from build123d import *

# Parameters (mm, degrees)
BOSS_EXTRUDE1_DEPTH = 2.5
CUT_EXTRUDE1_REACH  = 26.645
SKETCH2_R           = 1.715
SKETCH2_R_2         = 8.98
SKETCH3_R           = 2.6543
BOSS_EXTRUDE2_DEPTH = 70.305
BOSS_EXTRUDE3_START = 4
SKETCH4_R           = 21
SKETCH4_R_2         = 8.98
BOSS_EXTRUDE3_DEPTH = 4
SKETCH6_R           = 21
SKETCH6_R_2         = 8.98
BOSS_EXTRUDE4_DEPTH = 2
CUT_EXTRUDE3_START  = -15
SKETCH7_R           = 1.715
CUT_EXTRUDE3_DEPTH  = 15
SKETCH8_R           = 8.98
CUT_EXTRUDE4_DEPTH  = 2
SKETCH9_R           = 11.0744
SKETCH9_R_2         = 8.98
BOSS_EXTRUDE5_DEPTH = 2.35
BOSS_EXTRUDE6_REACH = 82.451
SKETCH10_R          = 12.48
SKETCH10_R_2        = 8.98
SKETCH12_R          = 21
SKETCH12_R_2        = 12.48
CUT_EXTRUDE5_DEPTH  = 57.805


with BuildPart() as part:
    # Sketch1 → Boss-Extrude1 (new body)
    with BuildSketch(Plane(origin=(0, 0, 0), x_dir=(1, 0, 0), z_dir=(0, 1, 0))):
        with BuildLine():
            Line((0.597960958, 12.236443242), (0.597960958, 17.5133))
            Line((0.597960958, 17.5133), (-2.819411684, 17.5133))
            Line((-2.819411684, 17.5133), (-2.819411684, 11.976881697))
            ThreePointArc((-2.819411684, 11.976881697), (-9.752212861, 8.278991937), (-13.533031252, 1.391065316))
            ThreePointArc((-13.533031252, 1.391065316), (-17.156497956, -0.999626805), (-13.683409812, -3.603965207))
            ThreePointArc((-13.683409812, -3.603965207), (-10.042516815, -11.01106651), (-2.819411684, -15.004561697))
            Line((-2.819411684, -15.004561697), (-2.819411684, -17.5133))
            Line((-2.819411684, -17.5133), (0.597960958, -17.5133))
            Line((0.597960958, -17.5133), (0.597960958, -15.264123242))
            ThreePointArc((0.597960958, -15.264123242), (9.161591247, -11.721092084), (13.538839655, -3.55233882))
            ThreePointArc((13.538839655, -3.55233882), (17.156522938, -1.000460972), (13.393344487, 1.331534062))
            ThreePointArc((13.393344487, 1.331534062), (8.853545908, 8.96396608), (0.597960958, 12.236443242))
        make_face()
    extrude(amount=BOSS_EXTRUDE1_DEPTH)

    # Sketch2 → Cut-Extrude1 (cut, up to next)
    with BuildSketch(Plane(origin=(0, 2.5, 0), x_dir=(1, 0, 0), z_dir=(0, 1, 0)), mode=Mode.PRIVATE) as cut_extrude1_sk1:
        with Locations(Location((-14.5034, -1.0795, 0), (0, 0, 270))):
            Circle(SKETCH2_R)
    cut_extrude1_tool1 = extrude(cut_extrude1_sk1.sketch, amount=-CUT_EXTRUDE1_REACH, mode=Mode.PRIVATE) & part.part
    # Sketch2 → Cut-Extrude1 (cut, up to next)
    with BuildSketch(Plane(origin=(0, 2.5, 0), x_dir=(1, 0, 0), z_dir=(0, 1, 0)), mode=Mode.PRIVATE) as cut_extrude1_sk2:
        with Locations(Location((14.5034, -1.0795, 0), (0, 0, 270))):
            Circle(SKETCH2_R)
    cut_extrude1_tool2 = extrude(cut_extrude1_sk2.sketch, amount=-CUT_EXTRUDE1_REACH, mode=Mode.PRIVATE) & part.part
    # Sketch2 → Cut-Extrude1 (cut, up to next)
    with BuildSketch(Plane(origin=(0, 2.5, 0), x_dir=(1, 0, 0), z_dir=(0, 1, 0)), mode=Mode.PRIVATE) as cut_extrude1_sk3:
        with Locations(Location((-0.0762, -1.51384, 0), (0, 0, 270))):
            Circle(SKETCH2_R_2)
    cut_extrude1_tool3 = extrude(cut_extrude1_sk3.sketch, amount=-CUT_EXTRUDE1_REACH, mode=Mode.PRIVATE) & part.part
    add(cut_extrude1_tool1.solids().sort_by_distance((-14.5034, 2.5, 1.0795))[0], mode=Mode.SUBTRACT)
    add(cut_extrude1_tool2.solids().sort_by_distance((14.5034, 2.5, 1.0795))[0], mode=Mode.SUBTRACT)
    add(cut_extrude1_tool3.solids().sort_by_distance((-0.0762, 2.5, 1.51384))[0], mode=Mode.SUBTRACT)

    # Sketch3 → Boss-Extrude2 (add)
    with BuildSketch(Plane(origin=(0, 2.5, 0), x_dir=(1, 0, 0), z_dir=(0, 1, 0))):
        with Locations(Location((-14.5034, -1.0795, 0), (0, 0, 68.556492541))):
            Circle(SKETCH3_R)
        with Locations(Location((14.5034, -1.0795, 0), (0, 0, 114.72164566))):
            Circle(SKETCH3_R)
    extrude(amount=BOSS_EXTRUDE2_DEPTH)

    # Sketch4 → Boss-Extrude3 (add)
    with BuildSketch(Plane(origin=(0, 72.805, 0), x_dir=(1, 0, 0), z_dir=(0, 1, 0)).offset(BOSS_EXTRUDE3_START)):
        with Locations(Location((-0.0762, -1.51384, 0), (0, 0, 270))):
            Circle(SKETCH4_R)
        with Locations(Location((-0.0762, -1.51384, 0), (0, 0, 270))):
            Circle(SKETCH4_R_2, mode=Mode.SUBTRACT)
    extrude(amount=-BOSS_EXTRUDE3_DEPTH)

    # Sketch6 → Boss-Extrude4 (add)
    with BuildSketch(Plane(origin=(0, 37.805, 0), x_dir=(-1, 0, 0), z_dir=(0, -1, 0))):
        with Locations(Location((0.0762, -1.51384, 0), (0, 0, 90))):
            Circle(SKETCH6_R)
        with Locations(Location((0.0762, -1.51384, 0), (0, 0, 270))):
            Circle(SKETCH6_R_2, mode=Mode.SUBTRACT)
    extrude(amount=BOSS_EXTRUDE4_DEPTH)

    # Sketch7 → Cut-Extrude3 (cut)
    with BuildSketch(Plane.XZ.offset(CUT_EXTRUDE3_START)):
        with Locations(Location((-14.5034, 1.0795, 0), (0, 0, 90))):
            Circle(SKETCH7_R)
        with Locations(Location((14.5034, 1.0795, 0), (0, 0, 90))):
            Circle(SKETCH7_R)
    extrude(amount=CUT_EXTRUDE3_DEPTH, mode=Mode.SUBTRACT)

    # Sketch8 → Cut-Extrude4 (cut)
    with BuildSketch(Plane(origin=(0, 76.805, 0), x_dir=(1, 0, 0), z_dir=(0, 1, 0))):
        with BuildLine():
            Line((-10.0762, -1.51384), (-7.3262, -15.51384))
            ThreePointArc((-7.3262, -15.51384), (-0.0762, -17.51384), (7.1738, -15.51384))
            Line((7.1738, -15.51384), (9.9238, -1.51384))
            Line((9.9238, -1.51384), (7.1738, 12.48616))
            ThreePointArc((7.1738, 12.48616), (-0.0762, 14.48616), (-7.3262, 12.48616))
            Line((-7.3262, 12.48616), (-10.0762, -1.51384))
        make_face()
        with Locations(Location((-0.0762, -1.51384, 0), (0, 0, 270))):
            Circle(SKETCH8_R, mode=Mode.SUBTRACT)
    extrude(amount=-CUT_EXTRUDE4_DEPTH, mode=Mode.SUBTRACT)

    # Sketch9 → Boss-Extrude5 (add)
    with BuildSketch(Plane.XZ):
        with Locations(Location((-0.0762, 1.51384, 0), (0, 0, 90))):
            Circle(SKETCH9_R)
        with Locations(Location((-0.0762, 1.51384, 0), (0, 0, 90))):
            Circle(SKETCH9_R_2, mode=Mode.SUBTRACT)
    extrude(amount=BOSS_EXTRUDE5_DEPTH)

    # Boss-Extrude6: up to this face of the body (flat: up to its plane)
    boss_extrude6_end = Plane(part.part.faces().sort_by_distance((-0.0762, 72.805, -18.892190304))[0])
    # Sketch10 → Boss-Extrude6 (add, up to the picked face)
    with BuildSketch(Plane(origin=(0, 2.5, 0), x_dir=(1, 0, 0), z_dir=(0, 1, 0)), mode=Mode.PRIVATE) as boss_extrude6_sk1:
        with Locations((-0.0762, -1.51384)):
            Circle(SKETCH10_R)
        with Locations(Location((-0.0762, -1.51384, 0), (0, 0, 270))):
            Circle(SKETCH10_R_2, mode=Mode.SUBTRACT)
    boss_extrude6_tool1 = split(extrude(boss_extrude6_sk1.sketch, amount=BOSS_EXTRUDE6_REACH, mode=Mode.PRIVATE), bisect_by=boss_extrude6_end, keep=Keep.BOTH, mode=Mode.PRIVATE)
    add(boss_extrude6_tool1.solids().sort_by(Axis((-12.203212, 2.5, 1.51384), (0, 1, 0)))[0])

    # Sketch12 → Cut-Extrude5 (cut)
    with BuildSketch(Plane.XZ.offset(-15)):
        with Locations(Location((-0.0762, 1.51384, 0), (0, 0, 90))):
            Circle(SKETCH12_R)
        with Locations(Location((-0.0762, 1.51384, 0), (0, 0, 189.400360909))):
            Circle(SKETCH12_R_2, mode=Mode.SUBTRACT)
    extrude(amount=-CUT_EXTRUDE5_DEPTH, mode=Mode.SUBTRACT)


solid = part.part
Source: CAD feature listing. Evaluate the final solid. Frame: model axes, mm. A direction names the side the tool comes from. Give positions to 0.01 mm unless a question says otherwise; leave off trailing zeros. Write each loop counter-clockwise with the first axis right and the second up, starting at its lowest first coordinate (ties: lowest second). Pieces come first, ordered by that corner, then holes. Notation, with made-up numbers: M 63.25,59 L 90.25,59 A14 ccw 90.25,79 Z; hole C -36,47.5 d3. An arc over 180 degrees is marked long. Return JSON: item names as keys, results as strings. Group by question number.
1) Ray query, L1, parallel to Z at x = 0, y = 2; L2, parallel to Y at x = -11.5, z = 9 (3 decimals); L3, parallel to Y at x = 14.5, z = -0.5 (3 decimals). Return the intervals inside material, ascending.
2) Draft query along Z for faces 1 (the face through (0.03, 75.819, -14.486)), 2 (the face through (-2, 2.5, 14)), 3 (the face through (-1, 1, 17.513)), 4 (the face through (-8.682, 75.819, -5.584)). Return one class per face: released by +Z, released by -Z, zero draft, split by the parting line, or undercut.
3) Cut plane A-A, the plane z = -6. Output: boundary loops of the cut face in (x, y) (3 decimals).
4) Cut plane B-B, the plane x = -1.5. Output: boundary loops of the cut face in (y, z) (3 decimals).
5) Cut plane D-D, the plane y = 23.5. Output: boundary loops of the cut face in (x, z), then the cut area to 3 significant figures.
6) Set-up query: faces 5 (the face through (0.598, 1, 16)), 6 (the face through (-3.403, -1.159, 12.077)), 7 (the face through (-2.819, 1, -15)), 8 (the face through (8.53, 75.82, 8.61)), 9 (the face through (6.232, 74.833, 21.544)). Return all of +Z, -Z, +X, -X, +Y, -Y with unobstructed straight access to the full face (end or side cutting, diameter ignored); none if empty.
7) First-contact query: pin 1 Ø6 at (x, y) = (-5.5, 23) entering from +Z; pin 2 Ø8 at (x, y) = (2, 42.5) entering from +Z; pin 3 Ø2 at (x, z) = (-10.5, -11.5) entering from -Y (3 decimals); pin 4 Ø11 at (x, z) = (-0.08, 1.51) entering from -Y. Flat tips, straight axial feed; report the tip coordinate or a pass-through.
8) Cut plane C-C, the plane y = 6. Output: boundary loops of the cut face in (x, z) (1 decimal).
Data:
{
 "1": {"L1": "z = -17.51 to -7.47, 10.49 to 17.51", "L2": "y = 0 to 2.5, 72.805 to 76.805", "L3": "y = 72.805 to 76.805"},
 "2": {"face 1": "undercut", "face 2": "zero draft", "face 3": "released by +Z", "face 4": "undercut"},
 "3": {"outline": "M -19.686,72.805 L -10.041,72.805 L -10.041,2.5 L -11.612,2.5 L -11.612,0 L -8.212,0 L -8.212,-2.35 L -4.994,-2.35 L -4.994,74.805 L -8.6,74.805 L -8.6,76.805 L -19.686,76.805 Z; M 4.841,-2.35 L 8.059,-2.35 L 8.059,0 L 11.459,0 L 11.459,2.5 L 9.888,2.5 L 9.888,72.805 L 19.534,72.805 L 19.534,76.805 L 8.448,76.805 L 8.448,74.805 L 4.841,74.805 Z"},
 "4": {"outline": "M -2.35,-9.469 L 0,-9.469 L 0,-17.513 L 2.5,-17.513 L 2.5,-10.885 L 72.805,-10.885 L 72.805,-19.438 L 76.805,-19.438 L 76.805,-14.414 L 74.805,-14.414 L 74.805,-7.353 L -2.35,-7.353 Z; M -2.35,10.38 L 74.805,10.38 L 74.805,17.442 L 76.805,17.442 L 76.805,22.466 L 72.805,22.466 L 72.805,13.912 L 2.5,13.912 L 2.5,17.513 L 0,17.513 L 0,12.496 L -2.35,12.496 Z"},
 "5": {"outline": "C -0.08,1.51 d24.96; hole C -0.08,1.51 d17.96", "area": "236 mm²"},
 "6": {"face 5": "+Z, +X, -Y", "face 6": "-Y", "face 7": "-Z, -X, -Y", "face 8": "+Y", "face 9": "+Y, -Y"},
 "7": {"pin 1": "stops at z = 13.76", "pin 2": "stops at z = 13.99", "pin 3": "stops at y = 72.805", "pin 4": "passes through"},
 "8": {"outline": "M -12.5,2.8 A2.7 ccw long -12.4,-0.5 A12.5 ccw 12.3,-0.3 A2.7 ccw long 12.4,2.6 A12.5 ccw Z; hole C -14.5,1.1 d3.4; hole C -0.1,1.5 d18; hole C 14.5,1.1 d3.4"}
}
